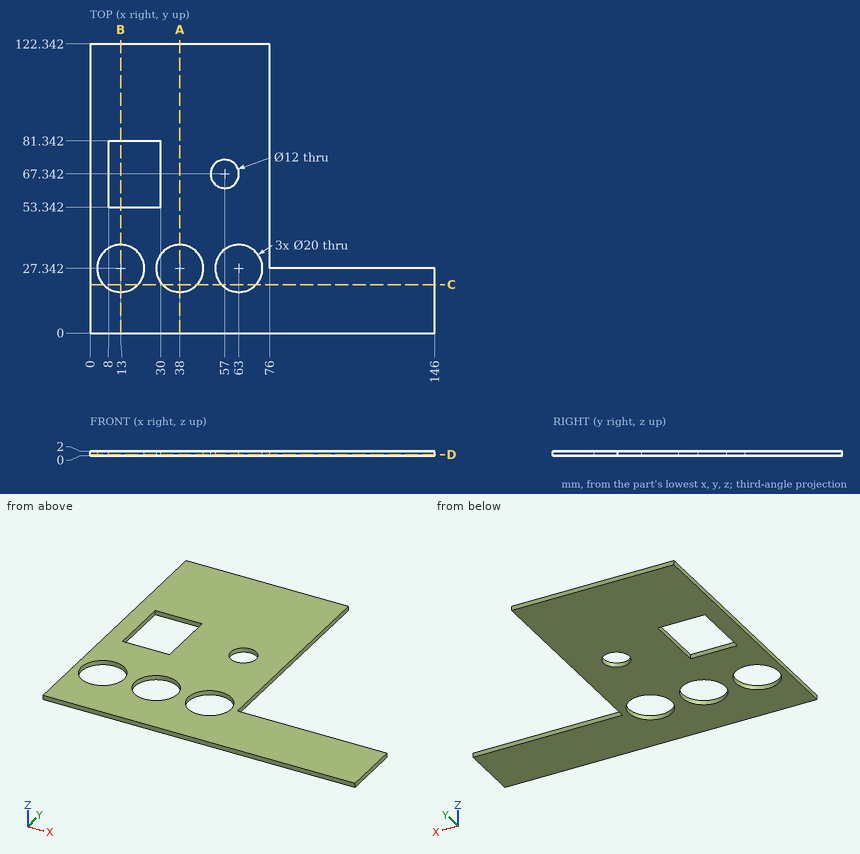
Geometry check sheet. Reference: drawing and pictorial views, mm from the part's lowest x, y, z. Coordinates: 2 decimals unless noted, no trailing zeros. Order: outer loops, then holes, each group sorted by start corner. A loop starts at its lowest first (then second) coordinate and runs counter-clockwise, first axis right, second up. Notation, with made-up numbers: (23.25, 28.25) -> (48.25, 28.25) arc R17 cw to (48.25, 39.25) -> close; hole circle Ø6 at (11, -31.75). An arc over 180 degrees is marked (long way). Put each result on its own line as item: value. Start each with the question number.
1) Cross-section at D-D (z = 0.5). Enter the section's corners in (x, y).
2) Cross-section at B-B (x = 13). Enter the section's corners in (y, z), plus the area to 3 significant figures.
3) Material ranges on L1, parallel to Y at x = 57, z = 1.3; L2, parallel to X at y = 59, z = 0.4; L3, parallel to Y at x = 9.5, z = 0.6, recorded low to high.
4) Cross-section at A-A (x = 38). Enter the section's corners in (y, z), plus the area to 3 significant figures.
5) Cross-section at C-C (y = 20.5). Enter the section's corners in (x, z).
Geometry check:
1. outline: (0, 0) -> (146, 0) -> (146, 27.34) -> (76, 27.34) -> (76, 122.34) -> (0, 122.34) -> close; hole circle Ø20 at (13, 27.34); hole (8, 53.34) -> (30, 53.34) -> (30, 81.34) -> (8, 81.34) -> close; hole circle Ø20 at (38, 27.34); hole circle Ø12 at (57, 67.34); hole circle Ø20 at (63, 27.34)
2. outline: (0, 0) -> (17.34, 0) -> (17.34, 2) -> (0, 2) -> close; (37.34, 0) -> (53.34, 0) -> (53.34, 2) -> (37.34, 2) -> close; (81.34, 0) -> (122.34, 0) -> (122.34, 2) -> (81.34, 2) -> close
2. area: 149 mm^2
3. L1: y = 0 to 19.34, 35.34 to 61.34, 73.34 to 122.34
3. L2: x = 0 to 8, 30 to 76
3. L3: y = 0 to 17.97, 36.71 to 53.34, 81.34 to 122.34
4. outline: (0, 0) -> (17.34, 0) -> (17.34, 2) -> (0, 2) -> close; (37.34, 0) -> (122.34, 0) -> (122.34, 2) -> (37.34, 2) -> close
4. area: 205 mm^2
5. outline: (0, 0) -> (5.71, 0) -> (5.71, 2) -> (0, 2) -> close; (20.29, 0) -> (30.71, 0) -> (30.71, 2) -> (20.29, 2) -> close; (45.29, 0) -> (55.71, 0) -> (55.71, 2) -> (45.29, 2) -> close; (70.29, 0) -> (146, 0) -> (146, 2) -> (70.29, 2) -> close
